Design review of the part built by this model. Coordinates are the model's own, in mm. Face numbers are marked on the shaded views. Give positions to 0.01 mm unless a question says otherwise; leave off trailing zeros. Order: outer loops, then holes, each group sorted by start corner. A loop starts at its lowest first (then second) coordinate and runs counter-clockwise, first axis right, second up. Notation, with made-up numbers: M -32,45 L -11,45 A24 cw -11,83 Z; hole C -17.5,31.5 d9. An arc over 180 degrees is marked long. Answer as a JSON object with one key per item and string values.
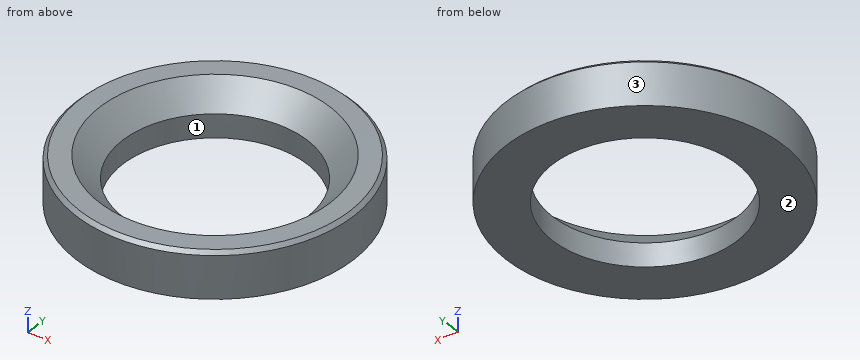
from build123d import *

# Parameters (mm, degrees)
F2_SIZE = 12.7
F3_SIZE = 2


with BuildPart() as f1:
    # F0 (on Front) → F1 (revolve)
    with BuildSketch(Plane.XZ):
        Polygon((50.756192, 25.59499), (50.800075, 0), (76.2, 0), (76.2, 25.4), align=None)
    revolve(axis=Axis((0, 0, 20.958871), (0, 0, 1)))

    # F2
    f2_edges = [f1.edges().sort_by_distance(p)[0] for p in [
        (-50.756192, 0, 25.59499),
    ]]
    chamfer(f2_edges, length=F2_SIZE)

    # F3
    f3_edges = [f1.edges().sort_by_distance(p)[0] for p in [
        (-76.2, 0, 25.4),
    ]]
    chamfer(f3_edges, length=F3_SIZE)


solid = f1.part
(1) Draft analysis for pull direction Y (two halves, no side actions). For the marked faces 1, 2 and 3, state which applies: +Y half, -Y half, draft (parallel to the pull), parting line (faces both ways), or undercut.
Checked values:
{"face 1": "undercut", "face 2": "draft", "face 3": "parting line"}
(2) Insertion check: pin 1 (10 mm diameter, centred on x = -4, z = 13.5, fed in from +Y); pin 2 (12 mm diameter, centred on x = -7, z = 18, fed in from -Y); pin 3 (1.5 mm diameter, centred on y = -27, z = 6, fed in from -X). Each pin has a flat end and moves straight along its axis. Give the tip position at first contact, or say it passes through.
Checked values:
{"pin 1": "stops at y = 76.2", "pin 2": "stops at y = -76.19", "pin 3": "stops at x = -71.54"}
(3) We need section A-A (z = 6). Write out the cut boundary in (x, y), plus the area to 3 significant figures.
Checked values:
{"outline": "C 0,0 d152.4; hole C 0,0 d101.58", "area": "10,100 mm^2"}
(4) To check wall thickness, follow L1, parallel to Z at x = 70, y = -16.5; L2, parallel to Y at x = -17.5, z = 18.5; L3, parallel to Y at x = -28.5, z = 20. State the ranges of each line that lie inside material, in increasing order. Write a range as from..to.
Checked values:
{"L1": "z = 0..25.43", "L2": "y = -74.16..-53.63, 53.63..74.16", "L3": "y = -70.67..-50.43, 50.43..70.67"}
